Check sheet for the drawn part. Datum: minimum x, y, z corner. Units: mm. A direction names the side the tool comes from. Give positions to 0.01 mm unless a question says otherwise; leave off trailing zeros. Order: outer loops, then holes, each group sorted by start corner. A loop starts at its lowest first (then second) coordinate and runs counter-clockwise, first axis right, second up. Notation, with made-up numbers: (-15, 79.5) -> (-8, 79.5) arc R21 ccw to (-8, 107.5) -> close; hole circle Ø3 at (63, 55.25). An arc over 180 degrees is marked (long way). Return JSON: item names as keys, results as strings. Group by question number.
(1) Release check for a two-part mould opening along Z. For the marked faces 1, 2 and 3 record: pulls with the +Z half, pulls with the -Z half, needs draft (parallel to the pull), parting line crosses it, or undercut.
(2) Thickness scan on line 1 along X through (y, z) = (22, 50); line 2 along Y through (x, z) = (13, 26); line 3 along Y through (x, z) = (69, 37.5). Record the ranges inside material, lowest first.
(3) Cross-section at A-A on z = 6.75. Enter the section's corners in (x, y), then the cut area to 3 significant figures.
(4) Depth check by flat-ended pin: pin 1 Ø9 at (x, z) = (92.75, 49.75) entering from +Y; pin 2 Ø6.5 at (x, z) = (6.75, 49.75) entering from +Y; pin 3 Ø9 at (x, z) = (49.75, 92.75) entering from -Y; pin 4 Ø13.5 at (x, z) = (41, 57.5) entering from -Y. Enter the tip coordinate at first touch or a pass-through.
(5) Cross-section at B-B on x = 92.75. Enter the section's corners in (y, z), then the cut area to 3 significant figures.
(6) Cross-section at C-C on x = 19. Enter the section's corners in (y, z).
(7) Tool access check on the marked faces 4, 5, 6 and 7. Record the directions out of +Z, -Z, +X, -X, +Y, -Y that give a thin tool (end or side, any length) a straight path to the whole face; none if there is none.
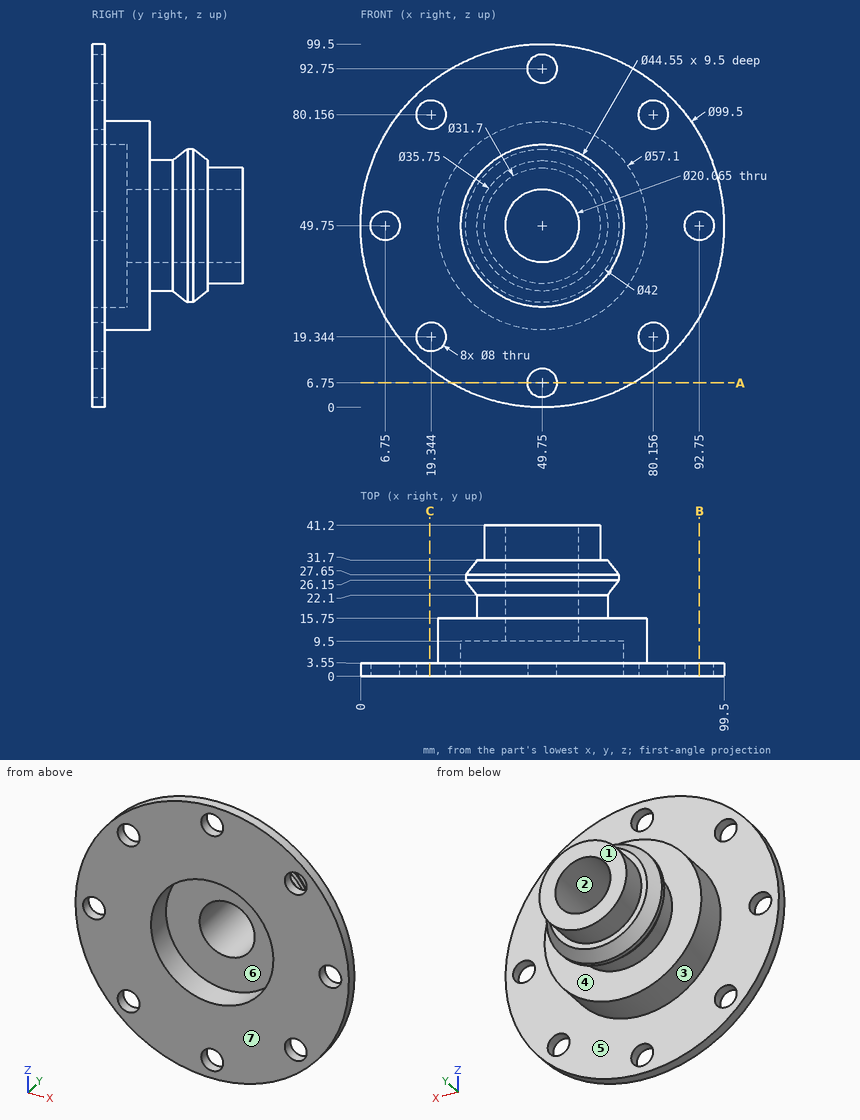
Verdict:
{
 "1": {"face 1": "needs draft", "face 2": "undercut", "face 3": "parting line crosses it"},
 "2": {"line 1": "31.88 to 39.72, 59.78 to 67.62", "line 2": "0 to 3.55", "line 3": "0 to 15.75"},
 "3": {"outline": "(24.73, 0) -> (45.75, 0) -> (45.75, 3.55) -> (24.73, 3.55) -> close; (53.75, 0) -> (74.77, 0) -> (74.77, 3.55) -> (53.75, 3.55) -> close", "area": "149 mm²"},
 "4": {"pin 1": "y = 3.55", "pin 2": "through", "pin 3": "y = 0", "pin 4": "y = 9.5"},
 "5": {"outline": "(0, 24.73) -> (3.55, 24.73) -> (3.55, 45.75) -> (0, 45.75) -> close; (0, 53.75) -> (3.55, 53.75) -> (3.55, 74.77) -> (0, 74.77) -> close", "area": "149 mm²"},
 "6": {"outline": "(0, 10.64) -> (3.55, 10.64) -> (3.55, 15.36) -> (0, 15.36) -> close; (0, 23.33) -> (3.55, 23.33) -> (3.55, 76.17) -> (0, 76.17) -> close; (0, 84.14) -> (3.55, 84.14) -> (3.55, 88.86) -> (0, 88.86) -> close"},
 "7": {"face 4": "none", "face 5": "+Y", "face 6": "-Y", "face 7": "+Z, -Z, +X, -X, -Y"}
}
